Source: CAD feature listing. Evaluate the final solid. Frame: model axes, mm. A direction names the side the tool comes from. Give positions to 0.01 mm unless a question says otherwise; leave off trailing zeros. Order: outer loops, then holes, each group sorted by start corner. A loop starts at its lowest first (then second) coordinate and runs counter-clockwise, first axis right, second up. Notation, with made-up numbers: (26, 14) - (70, 14) arc R14 cw to (70, 34) - close; hole circle Ø4 at (88, 20). An arc over 180 degrees is marked (long way). Write each question's results on one line, items separated by ' | '. Start each with the question number.
Item 1: Section D-D on y = 8. Output: boundary loops of the cut face in (x, z).
Item 2: Mould query, pull axis Y, two halves, no side actions, for faces 6 (the flat face through (50.218, 0, 5)), 7 (the flat face through (21, -17.5, 1)), 8 (the cylindrical face through (-3.88, -11.89, 1.01)). Classes: released by +Y, released by -Y, zero draft, split by the parting line, or undercut.
Item 3: Contact query for flat-ended pins moving along their axis: pin 1 Ø4 at (x, z) = (38.5, 11) entering from -Y; pin 2 Ø1 at (x, y) = (17, 11.5) entering from +Z; pin 3 Ø12.5 at (x, z) = (40.5, 10.5) entering from +Y. Output: stop coordinate, or through.
Item 4: Section B-B on x = 41.5. Output: boundary loops of the cut face in (y, z), and give its area (3 significant figures).
Item 5: Set-up query: faces 1 (the flat face through (-7.56, 0, 1)), 2 (the flat face through (43, 1, 9)), 3 (the flat face through (5, 10.575, 1)), 4 (the flat face through (43, -1, 9)), 5 (the flat face through (22, 17.5, 1)). Return all of +Z, -Z, +X, -X, +Y, -Y with unobstructed straight access to the full face (end or side cutting, diameter ignored); none if empty.
Item 6: Section C-C on z = 20.75. Output: boundary loops of the cut face in (x, y), and give its area (3 significant figures).
Item 7: Line query: line 1 along Y through (x, z) = (2, 1.75) (3 decimals); line 2 along Z through (x, y) = (5, -6); line 3 along Y through (x, z) = (46.5, 7.75). Output: solid intervals per line, ascending.
Item 8: Section A-A on x = 6.5. Output: boundary loops of the cut face in (y, z) (3 decimals).
Autodesk Inventor part; units mm, degrees
ref_plane "YZ Plane" through (0, 0, 0) normal (1, 0, 0) x (0, 1, 0)
ref_plane "XZ Plane" through (0, 0, 0) normal (0, 1, 0) x (-1, 0, 0)
ref_plane "XY Plane" through (0, 0, 0) normal (0, 0, 1) x (1, 0, 0)
ref_plane "Płaszczyzna konstrukcyjna1" through (3.373, 0, 0) normal (0, 0, 1) x (1, 0, 0)
sketch "Szkic1" plane through (3.373, 0, 0) normal (0, 0, 1) x (1, 0, 0)
  line L0 (-18.9331, -17.5) -> (46.8447, -17.5)
  line L1 (46.8447, -17.5) -> (46.8447, 17.5)
  line L2 (46.8447, 17.5) -> (-18.9331, 17.5)
  line L3 (-18.9331, 17.5) -> (-18.9331, -17.5)
  line L4 (-3.373, 0) -> (-37.9313, 0) construction
  line L5 (46.8447, 48.9998) -> (46.8447, 17.425) construction
  arc A0 (-19.7109, 13.5) -> (-19.7109, 10.5) centre (-19.7109, 12) ccw construction
  line L6 (-19.7109, 13.5) -> (-16.7109, 13.5) construction
  arc A1 (-16.7109, 10.5) -> (-16.7109, 13.5) centre (-16.7109, 12) ccw construction
  line L7 (-16.7109, 10.5) -> (-19.7109, 10.5) construction
  line L8 (-29.2109, -13.5) -> (-32.2109, -13.5) construction
  arc A2 (-32.2109, -10.5) -> (-32.2109, -13.5) centre (-32.2109, -12) ccw construction
  line L9 (-32.2109, -10.5) -> (-29.2109, -10.5) construction
  arc A3 (-29.2109, -13.5) -> (-29.2109, -10.5) centre (-29.2109, -12) ccw construction
  circle A4 centre (-16.7109, -12) radius 1.5 construction
  circle A5 centre (-32.2109, 12) radius 1.5 construction
  line L10 (-11.7109, 6.9) -> (-34.7109, 6.9) construction
  line L11 (-11.7109, -6.9) -> (-11.7109, 6.9) construction
  line L12 (-34.7109, -6.9) -> (-11.7109, -6.9) construction
  line L13 (-15.7109, -16) -> (-34.7109, -16) construction
  line L14 (-6.2109, -9.5) -> (-15.7109, -16) construction
  line L15 (-6.2109, 9.5) -> (-6.2109, -9.5) construction
  line L16 (-15.7109, 16) -> (-6.2109, 9.5) construction
  line L17 (-34.7109, 16) -> (-15.7109, 16) construction
  line L18 (-34.7109, -6.9) -> (-34.7109, -16)
  line L19 (-34.7109, 16) -> (-34.7109, 6.9)
  dimension "d0" = 35
extrude "Wyciągnięcie proste1" add sketch "Szkic1" along normal blind 2
sketch "Szkic2" plane through (0, 0, 0) normal (0, 1, 0) x (-1, 0, 0)
  line L0 (-50.2177, 2) -> (15.5601, 2)
  line L1 (-50.2177, 2) -> (-50.2177, 27)
  line L2 (-50.2177, 27) -> (-25.2177, 2)
  line L3 (-50.2177, 2) -> (-25.2177, 2)
  point P0 (0, 0)
  dimension "d3" = 25
  dimension "d4" = 25
extrude "Wyciągnięcie proste2" add sketch "Szkic2" along normal mid plane 2
sketch "Szkic3" plane through (3.373, 0, 2) normal (0, 0, 1) x (1, 0, 0)
  line L0 (-18.9331, 17.5) -> (-18.9331, -17.5)
  line L1 (-18.9331, -17.5) -> (-10.9331, -17.5)
  line L2 (-10.9331, -17.5) -> (-10.9331, 17.5)
  line L3 (-10.9331, 17.5) -> (-18.9331, 17.5)
  line L4 (-18.9331, 17.5) -> (-18.9331, -17.5)
  point P0 (-3.373, 0)
  dimension "d7" = 8
extrude "Wyciągnięcie proste3" cut sketch "Szkic3" against normal up to next
sketch "Szkic5" plane through (3.373, 0, 2) normal (0, 0, 1) x (1, 0, 0)
  circle A0 centre (-5.7553, 12.075) radius 1.5
  arc A1 (9.7447, 10.575) -> (9.7447, 13.575) centre (9.7447, 12.075) ccw
  arc A2 (6.7447, 13.575) -> (6.7447, 10.575) centre (6.7447, 12.075) ccw
  arc A3 (-2.7553, -13.425) -> (-2.7553, -10.425) centre (-2.7553, -11.925) ccw
  arc A4 (-5.7553, -10.425) -> (-5.7553, -13.425) centre (-5.7553, -11.925) ccw
  circle A5 centre (9.7447, -11.925) radius 1.5
  line L0 (-7.2553, -11.925) -> (11.2447, -11.925) construction
  line L1 (-5.7553, -13.425) -> (9.7447, -13.425)
  line L2 (9.7447, -10.425) -> (-5.7553, -10.425)
  arc A6 (-5.7553, -10.425) -> (-5.7553, -13.425) centre (-5.7553, -11.925) ccw
  arc A7 (9.7447, -13.425) -> (9.7447, -10.425) centre (9.7447, -11.925) ccw
  line L3 (-7.2553, 12.075) -> (11.2447, 12.075) construction
  line L4 (-5.7553, 10.575) -> (9.7447, 10.575)
  line L5 (9.7447, 13.575) -> (-5.7553, 13.575)
  arc A8 (-5.7553, 13.575) -> (-5.7553, 10.575) centre (-5.7553, 12.075) ccw
  arc A9 (9.7447, 10.575) -> (9.7447, 13.575) centre (9.7447, 12.075) ccw
  point P0 (-3.373, 0)
  point P1 (1.9947, -11.925)
  point P2 (1.9947, 12.075)
extrude "Wyciągnięcie proste5" cut sketch "Szkic5" against normal up to next
properties part number "hinge_support"
Evaluation:
1) outline: (-7.56, 0) - (50.22, 0) - (50.22, 2) - (-7.56, 2) - close
2) face 6: zero draft | face 7: released by -Y | face 8: undercut
3) pin 1: stops at y = -1 | pin 2: stops at z = 2 | pin 3: stops at y = 1
4) outline: (-17.5, 0) - (17.5, 0) - (17.5, 2) - (1, 2) - (1, 18.28) - (-1, 18.28) - (-1, 2) - (-17.5, 2) - close | area: 103 mm^2
5) face 1: +Z, -Z, -X, +Y, -Y | face 2: +Z, +X, -X, +Y | face 3: +Z, -Z | face 4: +Z, +X, -X, -Y | face 5: +Z, -Z, +X, -X, +Y
6) outline: (43.97, -1) - (50.22, -1) - (50.22, 1) - (43.97, 1) - close | area: 12.5 mm^2
7) line 1: y = -17.5 to -13.425, -10.425 to 10.575, 13.575 to 17.5 | line 2: z = 0 to 2 | line 3: y = -1 to 1
8) outline: (-17.5, 0) - (-13.425, 0) - (-13.425, 2) - (-17.5, 2) - close; (-10.425, 0) - (10.575, 0) - (10.575, 2) - (-10.425, 2) - close; (13.575, 0) - (17.5, 0) - (17.5, 2) - (13.575, 2) - close
